```python
from build123d import *

# Parameters (mm, degrees)
SKETCH1_R           = 9
BOSS_EXTRUDE1_DEPTH = 65
SKETCH2_R           = 0.5


with BuildPart() as part:
    # Sketch1 → Boss-Extrude1 (new body)
    with BuildSketch(Plane(origin=(0, 0, 0), x_dir=(1, 0, 0), z_dir=(0, 1, 0))):
        with Locations(Location((0, 0, 0), (0, 0, 270))):
            Circle(SKETCH1_R)
    extrude(amount=BOSS_EXTRUDE1_DEPTH)

    # Sketch2 → Cut-Revolve1 (revolve, cut)
    with BuildSketch(Plane(origin=(0, 0, 0), x_dir=(0, 0, -1), z_dir=(1, 0, 0))):
        with Locations((9, 62)):
            Circle(SKETCH2_R)
        Polygon((6.548746469, 65), (6.255894625, 64.46676314), (5.297470411, 64.46676314), (4.76423355, 65), align=None)
    revolve(axis=Axis((0, 0, 0), (0, 1, 0)), mode=Mode.SUBTRACT)


solid = part.part
```
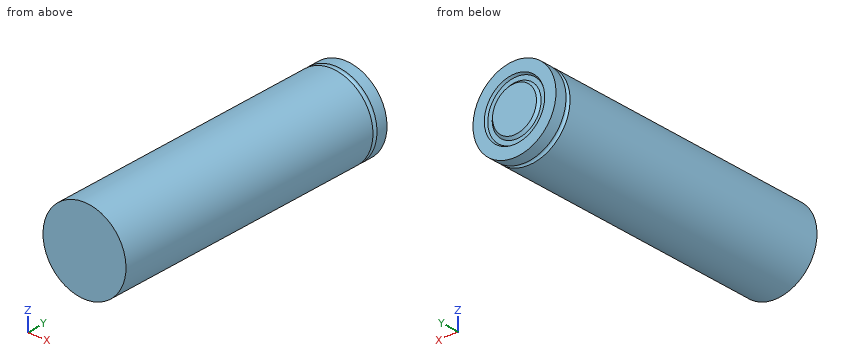
Geometry: final body of the model. Coordinates: model frame, mm. Give positions to 0.01 mm unless a question says otherwise; leave off trailing zeros. Loops run counter-clockwise (first coordinate to the right, second up) from the corner with the lowest first, then second, coordinate; pieces in that order, holes last. Notation, with made-up numbers: (-13, 72) - (26, 72) arc R29 ccw to (26, 99) - close; hole circle Ø3 at (-11.75, -13.5). An arc over 180 degrees is marked (long way). Answer as CSV lines item,"result". Start each with the question number.
(1) Ray query, line 1 along X through (y, z) = (39.5, -0.5); line 2 along Z through (x, y) = (-5, 49); line 3 along X through (y, z) = (9.5, 8.25). Return the intervals inside material, ascending. Write a range as [from, to].
(2) Section query A-A (y = 48.5). Output: boundary loops of the cut face in (x, z).
(3) Pin query (flat end, axial travel): P1, Ø8, axis at x = -4.5, y = 40.5, coming from the -Z side; P2, Ø2, axis at x = 6, y = 49.5, coming from the -Z side. Return the tip coordinate at first contact, or that it passes through.
Worked answers:
1,line 1,"x = [-8.99, 8.99]"
1,line 2,"z = [-7.48, 7.48]"
1,line 3,"x = [-3.6, 3.6]"
2,outline,"circle Ø18 at (0, 0)"
3,P1,"stops at z = -8.99"
3,P2,"stops at z = -7.48"
